Here's how the part is built. I have some questions about the finished solid (model axes, mm). A direction names the side the tool comes from. Give positions to 0.01 mm unless a question says otherwise; leave off trailing zeros. Order: outer loops, then holes, each group sorted by start corner. A loop starts at its lowest first (then second) coordinate and runs counter-clockwise, first axis right, second up.
Autodesk Inventor part; units mm, degrees
ref_plane "YZ Plane" through (0, 0, 0) normal (1, 0, 0) x (0, 1, 0)
ref_plane "XZ Plane" through (0, 0, 0) normal (0, 1, 0) x (-1, 0, 0)
ref_plane "XY Plane" through (0, 0, 0) normal (0, 0, 1) x (1, 0, 0)
sketch "スケッチ1" plane through (0, 0, 0) normal (0, 0, 1) x (1, 0, 0)
  line L0 (-25.3, 21.7) -> (25.3, 21.7)
  line L1 (25.3, 21.7) -> (25.3, -21.7)
  line L2 (25.3, -21.7) -> (-25.3, -21.7)
  line L3 (-25.3, -21.7) -> (-25.3, 21.7)
  circle A0 centre (-22.1, 18.5) radius 1.6
  circle A1 centre (22.1, 18.5) radius 1.6
  circle A2 centre (22.1, -18.5) radius 1.6
  circle A3 centre (-22.1, -18.5) radius 1.6
  line L4 (-18.1, 19.2) -> (-18.1, 14.5)
  line L5 (-18.1, 14.5) -> (-22.8, 14.5)
  line L6 (-22.8, 14.5) -> (-22.8, -14.5)
  line L7 (-22.8, -14.5) -> (-18.1, -14.5)
  line L8 (-18.1, -14.5) -> (-18.1, -19.2)
  line L9 (-18.1, -19.2) -> (18.1, -19.2)
  line L10 (18.1, -19.2) -> (18.1, -14.5)
  line L11 (18.1, -14.5) -> (22.8, -14.5)
  line L12 (22.8, -14.5) -> (22.8, 14.5)
  line L13 (22.8, 14.5) -> (18.1, 14.5)
  line L14 (18.1, 14.5) -> (18.1, 19.2)
  line L15 (18.1, 19.2) -> (-18.1, 19.2)
  point P0 (0, 0)
  point P1 (0, 21.7)
  point P2 (-25.3, 0)
  dimension "d0" = 50.6
  dimension "d1" = 43.4
  dimension "d2" = 3.2
  dimension "d3" = 44.2
  dimension "d4" = 37
  dimension "d5" = 22.1
  dimension "d6" = 18.5
  dimension "d7" = 2.5
  dimension "d8" = 2.5
  dimension "d9" = 2.5
  dimension "d10" = 2.5
  dimension "d11" = 4
  dimension "d12" = 4
  dimension "d13" = 4
  dimension "d14" = 4
  dimension "d15" = 4
extrude "押し出し1" add sketch "スケッチ1" along normal blind 1.5
sketch "スケッチ2" plane through (0, 0, 0) normal (0, 0, -1) x (-1, 0, 0)
  line L0 (-25.3, 21.7) -> (25.3, 21.7)
  line L1 (-25.3, -21.7) -> (-25.3, 21.7)
  circle A0 centre (-22.1, 18.5) radius 1.6
  line L2 (25.3, -21.7) -> (-25.3, -21.7)
  circle A1 centre (-22.1, -18.5) radius 1.6
  circle A2 centre (22.1, -18.5) radius 1.6
  line L3 (25.3, 21.7) -> (25.3, -21.7)
  circle A3 centre (22.1, 18.5) radius 1.6
  point P0 (0, 0)
extrude "押し出し2" add sketch "スケッチ2" along normal blind 1.5
sketch "スケッチ3" plane through (-25.3, 21.7, 1.5) normal (0, 1, 0) x (1, 0, 0)
  line L0 (0, 3) -> (0, 0)
  line L1 (50.6, 0) -> (0, 0)
  line L2 (50.6, 3) -> (50.6, 0)
  line L3 (0, 3) -> (50.6, 3)
  point P0 (25.3, 1.5)
extrude "押し出し3" add sketch "スケッチ3" along normal blind 3.6
sketch "スケッチ4" plane through (-25.3, -21.7, 1.5) normal (0, -1, 0) x (1, 0, 0)
  line L0 (50.6, -3) -> (50.6, 0)
  line L1 (0, 0) -> (50.6, 0)
  line L2 (0, 0) -> (0, -3)
  line L3 (50.6, -3) -> (0, -3)
  point P0 (25.3, -1.5)
extrude "押し出し4" add sketch "スケッチ4" along normal blind 3.6
equation "\"d8\" = d7"
equation "\"d9\" = d7"
equation "\"d10\" = d7"
equation "\"d12\" = d11"
equation "\"d13\" = d11"
equation "\"d14\" = d11"
equation "\"d15\" = d11"
properties part number "fan_controller_case_bottom"
Q1. If we section it at A-A on y = 18.5: List the corners of the cut face in (x, z) for me, plus the area to 3 significant figures.
Filled sheet:
outline: (-25.3, -1.5) - (-23.7, -1.5) - (-23.7, 1.5) - (-25.3, 1.5) - close; (-20.5, -1.5) - (20.5, -1.5) - (20.5, 1.5) - (18.1, 1.5) - (18.1, 0) - (-18.1, 0) - (-18.1, 1.5) - (-20.5, 1.5) - close; (23.7, -1.5) - (25.3, -1.5) - (25.3, 1.5) - (23.7, 1.5) - close
area: 78.3 mm2
Q2. For faces 1 (the face through (0, -25.3, 0)), 2 (the face through (0, -19.2, 1)), which set-ups out of +Z, -Z, +X, -X, +Y, -Y let a thin tool reach every point of the face, with its end or its side?
Filled sheet:
face 1: +Z, -Z, +X, -X, -Y
face 2: +Z
Q3. I'm going to push flat-ended pins straight in: P1, Ø1, axis at x = 1, y = -6, coming from the +Z side; P2, Ø4, axis at x = 22.1, y = -18.5, coming from the -Z side. Where does each tip first touch, or does it pass through?
Filled sheet:
P1: stops at z = 0
P2: stops at z = -1.5
Q4. If we section it at D-D on x = 16.5: List the corners of the cut face in (y, z) for me.
Filled sheet:
outline: (-25.3, -1.5) - (25.3, -1.5) - (25.3, 1.5) - (19.2, 1.5) - (19.2, 0) - (-19.2, 0) - (-19.2, 1.5) - (-25.3, 1.5) - close
Q5. If we section it at B-B on x = -22.1: List the corners of the cut face in (y, z) for me, plus the area to 3 significant figures.
Filled sheet:
outline: (-25.3, -1.5) - (-20.1, -1.5) - (-20.1, 1.5) - (-25.3, 1.5) - close; (-16.9, -1.5) - (16.9, -1.5) - (16.9, 1.5) - (14.5, 1.5) - (14.5, 0) - (-14.5, 0) - (-14.5, 1.5) - (-16.9, 1.5) - close; (20.1, -1.5) - (25.3, -1.5) - (25.3, 1.5) - (20.1, 1.5) - close
area: 89.1 mm2
Q6. Thinking about a two-plate mould opening in Y: for faces 3 (the face through (0, 25.3, 0)), 4 (the face through (25.3, 0, 0)), 5 (the face through (-18.1, -17, 1)), which applies, released by +Y, released by -Y, zero draft, split by the parting line, or undercut?
Filled sheet:
face 3: released by +Y
face 4: zero draft
face 5: undercut
Q7. If we section it at C-C on z = 1.05: List the corners of the cut face in (x, y) for me.
Filled sheet:
outline: (-25.3, -25.3) - (25.3, -25.3) - (25.3, 25.3) - (-25.3, 25.3) - close; hole circle Ø3.2 at (-22.1, -18.5); hole circle Ø3.2 at (-22.1, 18.5); hole (-22.8, -14.5) - (-18.1, -14.5) - (-18.1, -19.2) - (18.1, -19.2) - (18.1, -14.5) - (22.8, -14.5) - (22.8, 14.5) - (18.1, 14.5) - (18.1, 19.2) - (-18.1, 19.2) - (-18.1, 14.5) - (-22.8, 14.5) - close; hole circle Ø3.2 at (22.1, -18.5); hole circle Ø3.2 at (22.1, 18.5)
Q8. I need wall thicknesses on L1, parallel to X at y = -18.5, z = 0.6; L2, parallel to Y at x = 22.1, z = 0.65; L3, parallel to Y at x = -22.1, z = -0.65. Which ranges of each line are inside material? Lowest first, please.
Filled sheet:
L1: x = -25.3 to -23.7, -20.5 to -18.1, 18.1 to 20.5, 23.7 to 25.3
L2: y = -25.3 to -20.1, -16.9 to -14.5, 14.5 to 16.9, 20.1 to 25.3
L3: y = -25.3 to -20.1, -16.9 to 16.9, 20.1 to 25.3
